Input: part model. Units: mm. Frame: model coordinates. A direction names the side the tool comes from. Give positions to 0.01 mm unless a question says otherwise; leave off trailing zeros. Write each loop counter-clockwise with the first axis right and the second up, starting at its lowest first coordinate (ties: lowest second). Pieces come first, ordered by that corner, then holes. Notation, with made-up numbers: (-30, -35) -> (-26, -35) arc R26 cw to (-26, -14) -> close; hole circle Ø5 at (15, 18.25). An arc over 180 degrees is marked (long way). Return JSON: item names as keys, results as strings. Group by question number.
Item 1: Pin query (flat end, axial travel): P1, Ø1, axis at y = 1, z = 21, coming from the +X side; P2, Ø1.6, axis at x = -23, y = 2, coming from the +Z side; P3, Ø1.5, axis at y = 1.5, z = -11.5, coming from the -X side. Return the tip coordinate at first contact, or that it passes through.
Item 2: Section D-D, the plane y = 2.55. Count the separate pieces of the cut face and the enclosed holes in it, then the cut area to 3 significant figures.
Item 3: Section A-A, the plane z = 0. Return loops of the section in (x, y) (3 decimals).
Item 4: Section C-C, the plane z = -7. Return loops of the section in (x, y) (3 decimals).
Item 5: Line query: line 1 (X direction, y = 2.25, z = 0); line 2 (X direction, y = 1.05, z = -22) (3 decimals). Output: solid intervals per line, ascending. Write a range as [from, to].
Item 6: Section B-B, the plane x = 35. Return loops of the section in (y, z) (3 decimals).
Item 7: Set-up query: faces 5 (the face through (-22, 2, 15.8)), 6 (the face through (-41.2, 2, 0)), 7 (the face through (28.5, 2, -13)), 8 (the face through (28.5, 2, 13)), 9 (the face through (-21, 2, 3.175)). Return all of +Z, -Z, +X, -X, +Y, -Y with unobstructed straight access to the full face (end or side cutting, diameter ignored); none if empty.
Item 8: Mould query, pull axis X, two halves, no side actions, for faces 1 (the face through (3.175, 2, -21)), 2 (the face through (41.2, 2, 0)), 3 (the face through (-3.175, 2, -21)), 4 (the face through (22, 2, 15.8)). Classes: released by +X, released by -X, zero draft, split by the parting line, or undercut.
from build123d import *

# Parameters (mm, degrees)
SKETCH1_R           = 2.54
BOSS_EXTRUDE1_DEPTH = 3.175


with BuildPart() as part:
    # Sketch1 → Boss-Extrude1 (new body)
    with BuildSketch(Plane(origin=(0, 0, 0), x_dir=(1, 0, 0), z_dir=(0, 1, 0))):
        with BuildLine():
            Line((15.7999938, -28.4999938), (-15.7999938, -28.4999938))
            Line((-15.7999938, -28.4999938), (-15.7999938, -15.7999938))
            Line((-15.7999938, -15.7999938), (-28.4999938, -15.7999938))
            Line((-28.4999938, -15.7999938), (-28.4999938, -9.525))
            Line((-28.4999938, -9.525), (-36.1199938, -9.525))
            ThreePointArc((-36.1199938, -9.525), (-39.712096248, -8.037102448), (-41.1999938, -4.445))
            Line((-41.1999938, -4.445), (-41.1999938, 4.445))
            ThreePointArc((-41.1999938, 4.445), (-39.712096248, 8.037102448), (-36.1199938, 9.525))
            Line((-36.1199938, 9.525), (-28.4999938, 9.525))
            Line((-28.4999938, 9.525), (-28.4999938, 15.7999938))
            Line((-28.4999938, 15.7999938), (-15.7999938, 15.7999938))
            Line((-15.7999938, 15.7999938), (-15.7999938, 28.4999938))
            Line((-15.7999938, 28.4999938), (15.7999938, 28.4999938))
            Line((15.7999938, 28.4999938), (15.7999938, 15.7999938))
            Line((15.7999938, 15.7999938), (28.4999938, 15.7999938))
            Line((28.4999938, 15.7999938), (28.4999938, 9.525))
            Line((28.4999938, 9.525), (36.1199938, 9.525))
            ThreePointArc((36.1199938, 9.525), (39.712096248, 8.037102448), (41.1999938, 4.445))
            Line((41.1999938, 4.445), (41.1999938, -4.445))
            ThreePointArc((41.1999938, -4.445), (39.712096248, -8.037102448), (36.1199938, -9.525))
            Line((36.1199938, -9.525), (28.4999938, -9.525))
            Line((28.4999938, -9.525), (28.4999938, -15.7999938))
            Line((28.4999938, -15.7999938), (15.7999938, -15.7999938))
            Line((15.7999938, -15.7999938), (15.7999938, -28.4999938))
        make_face()
        with Locations((-34.8499938, 0)):
            Circle(SKETCH1_R, mode=Mode.SUBTRACT)
        with Locations((34.8499938, 0)):
            Circle(SKETCH1_R, mode=Mode.SUBTRACT)
        with BuildLine():
            Line((-18.783553311, 3.175), (-22.86, 3.175))
            Line((-22.86, 3.175), (-22.86, -3.175))
            Line((-22.86, -3.175), (-18.783553311, -3.175))
            ThreePointArc((-18.783553311, -3.175), (-13.470384182, -13.470384182), (-3.175, -18.783553311))
            Line((-3.175, -18.783553311), (-3.175, -22.86))
            Line((-3.175, -22.86), (3.175, -22.86))
            Line((3.175, -22.86), (3.175, -18.783553311))
            ThreePointArc((3.175, -18.783553311), (13.470384182, -13.470384182), (18.783553311, -3.175))
            Line((18.783553311, -3.175), (22.86, -3.175))
            Line((22.86, -3.175), (22.86, 3.175))
            Line((22.86, 3.175), (18.783553311, 3.175))
            ThreePointArc((18.783553311, 3.175), (13.470384182, 13.470384182), (3.175, 18.783553311))
            Line((3.175, 18.783553311), (3.175, 22.86))
            Line((3.175, 22.86), (-3.175, 22.86))
            Line((-3.175, 22.86), (-3.175, 18.783553311))
            ThreePointArc((-3.175, 18.783553311), (-13.470384182, 13.470384182), (-18.783553311, 3.175))
        make_face(mode=Mode.SUBTRACT)
    extrude(amount=BOSS_EXTRUDE1_DEPTH)


solid = part.part
Answer below:
{
 "1": {"P1": "stops at x = 15.8", "P2": "stops at z = 15.8", "P3": "stops at x = -28.5"},
 "2": {"separate pieces": "1", "enclosed holes": "3", "area": "1,790 mm2"},
 "3": {"outline": "(-41.2, 0) -> (-37.39, 0) -> (-37.39, 3.175) -> (-41.2, 3.175) -> close; (-32.31, 0) -> (-22.86, 0) -> (-22.86, 3.175) -> (-32.31, 3.175) -> close; (22.86, 0) -> (32.31, 0) -> (32.31, 3.175) -> (22.86, 3.175) -> close; (37.39, 0) -> (41.2, 0) -> (41.2, 3.175) -> (37.39, 3.175) -> close"},
 "4": {"outline": "(-40.511, 0) -> (-17.717, 0) -> (-17.717, 3.175) -> (-40.511, 3.175) -> close; (17.717, 0) -> (40.511, 0) -> (40.511, 3.175) -> (17.717, 3.175) -> close"},
 "5": {"line 1": "x = [-41.2, -37.39], [-32.31, -22.86], [22.86, 32.31], [37.39, 41.2]", "line 2": "x = [-15.8, -3.175], [3.175, 15.8]"},
 "6": {"outline": "(0, -9.525) -> (3.175, -9.525) -> (3.175, -2.536) -> (0, -2.536) -> close; (0, 2.536) -> (3.175, 2.536) -> (3.175, 9.525) -> (0, 9.525) -> close"},
 "7": {"face 5": "+Z, -X, +Y, -Y", "face 6": "+Z, -Z, -X, +Y, -Y", "face 7": "-Z, +X, +Y, -Y", "face 8": "+Z, +X, +Y, -Y", "face 9": "+Y, -Y"},
 "8": {"face 1": "undercut", "face 2": "released by +X", "face 3": "undercut", "face 4": "zero draft"}
}
